```python
from build123d import *

# Parameters (mm, degrees)
SKETCH1_W               = 235
SKETCH1_H               = 10
BOSS_EXTRUDE1_DEPTH     = 160
CUT_EXTRUDE1_DEPTH      = 7
SKETCH5_R               = 5
CUT_EXTRUDE2_DEPTH      = 33
SKETCH6_R               = 2.05
CUT_EXTRUDE3_DEPTH      = 33
ENL_V_MAT_EXTRU_2_DEPTH = 10
ENL_V_MAT_EXTRU_3_DEPTH = 10


with BuildPart() as part:
    # Sketch1 → Boss-Extrude1 (new body)
    with BuildSketch(Plane.XY):
        with Locations((117.5, 5)):
            Rectangle(SKETCH1_W, SKETCH1_H)
    extrude(amount=BOSS_EXTRUDE1_DEPTH)

    # Sketch3 → Cut-Extrude1 (cut)
    with BuildSketch(Plane.XZ):
        with BuildLine():
            Line((137.5, 132), (137.5, 82))
            ThreePointArc((137.5, 82), (157.5, 62), (177.5, 82))
            Line((177.5, 82), (177.5, 132))
            ThreePointArc((177.5, 132), (157.5, 152), (137.5, 132))
        make_face()
        with BuildLine():
            Line((57.5, 132), (57.5, 82))
            ThreePointArc((57.5, 82), (77.5, 62), (97.5, 82))
            Line((97.5, 82), (97.5, 132))
            ThreePointArc((97.5, 132), (77.5, 152), (57.5, 132))
        make_face()
    extrude(amount=-CUT_EXTRUDE1_DEPTH, mode=Mode.SUBTRACT)

    # Sketch5 → Cut-Extrude2 (cut)
    with BuildSketch(Plane.XZ.offset(-7)):
        with Locations(Location((77.5, 107, 0), (0, 0, 270))):
            Circle(SKETCH5_R)
        with Locations((157.5, 107)):
            Circle(SKETCH5_R)
    extrude(amount=-CUT_EXTRUDE2_DEPTH, mode=Mode.SUBTRACT)

    # Sketch6 → Cut-Extrude3 (cut)
    with BuildSketch(Plane.XZ.offset(-7)):
        with Locations(Location((77.5, 82, 0), (0, 0, 270))):
            Circle(SKETCH6_R)
        with Locations((77.5, 132)):
            Circle(SKETCH6_R)
        with Locations((157.5, 82)):
            Circle(SKETCH6_R)
        with Locations(Location((157.5, 132, 0), (0, 0, 270))):
            Circle(SKETCH6_R)
    extrude(amount=-CUT_EXTRUDE3_DEPTH, mode=Mode.SUBTRACT)

    # Esquisse2 → Enlèv. mat.-Extru.2 (cut)
    with BuildSketch(Plane.XZ):
        Polygon((0, 135), (10, 135), (10, 136.55), (15.5, 136.55), (15.5, 135), (21.5, 135), (21.5, 131), (15.5, 131), (15.5, 129.45), (10, 129.45), (10, 131), (0, 131), align=None)
        Polygon((0, 29), (10, 29), (10, 30.55), (15.5, 30.55), (15.5, 29), (21.5, 29), (21.5, 25), (15.5, 25), (15.5, 23.45), (10, 23.45), (10, 25), (0, 25), align=None)
        Polygon((235, 25), (225, 25), (225, 23.45), (219.5, 23.45), (219.5, 25), (213.5, 25), (213.5, 29), (219.5, 29), (219.5, 30.55), (225, 30.55), (225, 29), (235, 29), align=None)
        Polygon((235, 131), (225, 131), (225, 129.45), (219.5, 129.45), (219.5, 131), (213.5, 131), (213.5, 135), (219.5, 135), (219.5, 136.55), (225, 136.55), (225, 135), (235, 135), align=None)
    extrude(amount=-ENL_V_MAT_EXTRU_2_DEPTH, mode=Mode.SUBTRACT)

    # Esquisse3 → Enlèv. mat.-Extru.3 (cut)
    with BuildSketch(Plane.XZ):
        Polygon((49, 160), (49, 150), (50.55, 150), (50.55, 144.5), (49, 144.5), (49, 138.5), (45, 138.5), (45, 144.5), (43.45, 144.5), (43.45, 150), (45, 150), (45, 160), align=None)
        Polygon((190, 138.5), (186, 138.5), (186, 144.5), (184.45, 144.5), (184.45, 150), (186, 150), (186, 160), (190, 160), (190, 150), (191.55, 150), (191.55, 144.5), (190, 144.5), align=None)
        Polygon((186, 0), (186, 10), (184.45, 10), (184.45, 15.5), (186, 15.5), (186, 21.5), (190, 21.5), (190, 15.5), (191.55, 15.5), (191.55, 10), (190, 10), (190, 0), align=None)
        Polygon((45, 21.5), (49, 21.5), (49, 15.5), (50.55, 15.5), (50.55, 10), (49, 10), (49, 0), (45, 0), (45, 10), (43.45, 10), (43.45, 15.5), (45, 15.5), align=None)
    extrude(amount=-ENL_V_MAT_EXTRU_3_DEPTH, mode=Mode.SUBTRACT)


solid = part.part
```
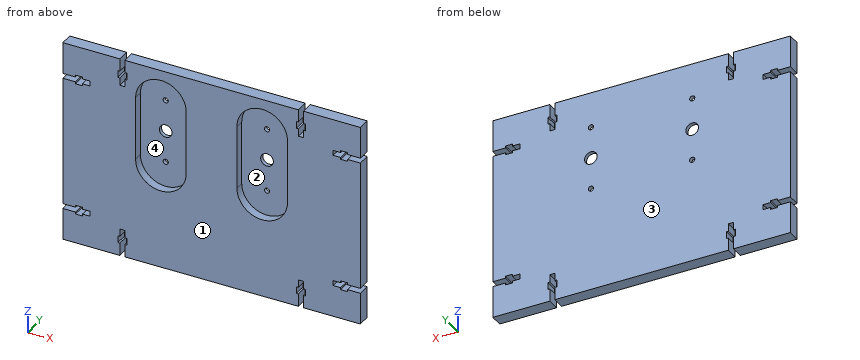
Here's how the part is built. I have some questions about the finished solid (model axes, mm). Face numbers are marked on the shaded views. A direction names the side the tool comes from. Coordinates: 2 decimals unless noted, no trailing zeros. Order: outer loops, then holes, each group sorted by start corner. A loop starts at its lowest first (then second) coordinate and runs counter-clockwise, first axis right, second up. Notation, with made-up numbers: M 31,-10 L 87,-10 A22 cw 87,29 Z; hole C -4.5,31 d4. An arc over 180 degrees is marked long. Answer as a JSON object with one key per item and string values. Group by question number.
(1) If we mould it in two halves opening along Z, with no side actions, what happens to the marked faces 1 and 2? For each: released by +Z, released by -Z, zero draft, split by the parting line, or undercut.
(2) Suppose I cut it at A-A, the plane z = 107. Please give me the cut outline in (x, y).
(3) Which directions (+Z, -Z, +X, -X, +Y, -Y) give clear straight access to the entire face, cutting with the end or side of a thin tool? Please do the marked faces 3 and 4.
(4) Suppose I cut it at D-D, the plane z = 65.5. Please give me the cut outline in (x, y), then the cut area to 3 significant figures.
(5) Suppose I cut it at C-C, the plane y = 5.5. State how many separate pieces and enclosed holes the cut face has, then the cut area to 3 significant figures.
(6) For pin 1 (10 mm diameter, centred on x = 68.5, z = 91.5, fed in from -Y), with a flat end and sliding along its axis, tell me the tip position at first contact or that it passes through.
(7) Suppose I cut it at B-B, the plane x = 86.5. Please give me the cut outline in (y, z), then the cut area to 4 significant figures.
(8) I need wall thicknesses on probe 1 along X at (y, z) = (8.6, 132); probe 2 along Z at (x, y) = (157.5, 8.05); probe 3 along X at (y, z) = (2.5, 7.5). Which ranges of each line are inside material? Lowest first, please.
Values found:
{
 "1": {"face 1": "zero draft", "face 2": "undercut"},
 "2": {"outline": "M 0,0 L 57.5,0 L 57.5,7 L 72.5,7 L 72.5,10 L 0,10 Z; M 82.5,7 L 97.5,7 L 97.5,0 L 137.5,0 L 137.5,7 L 152.5,7 L 152.5,10 L 82.5,10 Z; M 162.5,7 L 177.5,7 L 177.5,0 L 235,0 L 235,10 L 162.5,10 Z"},
 "3": {"face 3": "+Z, -Z, +X, -X, +Y", "face 4": "-Y"},
 "4": {"outline": "M 0,0 L 66.2,0 L 66.2,7 L 88.8,7 L 88.8,0 L 146.2,0 L 146.2,7 L 168.8,7 L 168.8,0 L 235,0 L 235,10 L 0,10 Z", "area": "2,030 mm^2"},
 "5": {"separate pieces": "1", "enclosed holes": "2", "area": "30,300 mm^2"},
 "6": {"pin 1": "stops at y = 7"},
 "7": {"outline": "M 0,0 L 10,0 L 10,160 L 0,160 L 0,149.86 L 7,149.86 L 7,64.14 L 0,64.14 Z", "area": "1,000 mm^2"},
 "8": {"probe 1": "x = 21.5 to 75.45, 79.55 to 155.45, 159.55 to 213.5", "probe 2": "z = 0 to 79.95, 84.05 to 102, 112 to 129.95, 134.05 to 160", "probe 3": "x = 0 to 45, 49 to 186, 190 to 235"}
}
